Verification items for the finished model (mm, model axes). Give positions to 0.01 mm unless a question says otherwise; leave off trailing zeros. Write each loop counter-clockwise with the first axis right and the second up, starting at its lowest first coordinate (ties: lowest second). Pieces come first, ordered by that corner, then holes.
from build123d import *

# Parameters (mm, degrees)
EXTRUDE002_DEPTH = 3


with BuildPart() as axle_hex_extrude:
    # Sketch009 → Extrude002 (new body)
    with BuildSketch(Plane.YZ.offset(31)):
        Polygon((-48.5, -42.556624), (-51, -41.113249), (-53.5, -42.556624), (-53.5, -45.443376), (-51, -46.886751), (-48.5, -45.443376), align=None)
    extrude(amount=-EXTRUDE002_DEPTH)


with BuildPart() as axle_front:
    # Sketch008 → Revolve001 (revolve)
    with BuildSketch(Plane.XZ.offset(51)):
        with BuildLine():
            Line((27.5, -42.5), (-27.5, -42.5))
            Line((-27.5, -42.5), (-27.5, -37))
            Line((-27.5, -37), (-28, -37))
            ThreePointArc((-28, -37), (-29.86452, -40.281569), (-30.511358, -44))
            Line((-30.511358, -44), (30.511358, -44))
            ThreePointArc((30.511358, -44), (30.236308, -40.148184), (28, -37))
            Line((27.5, -37), (28, -37))
            Line((27.5, -42.5), (27.5, -37))
        make_face()
    revolve(axis=Axis((2, -51, -44), (1, 0, 0)))

    # Cut: cut axle-hex-extrude
    add(axle_hex_extrude.part, mode=Mode.SUBTRACT)


with BuildPart() as axle_back:
    # Part__Mirroring001: instance of axle-front
    add(axle_front.part.mirror(Plane(origin=(0, 0, 0), x_dir=(1, 0, 0), z_dir=(0, 1, 0))))


solid = axle_back.part
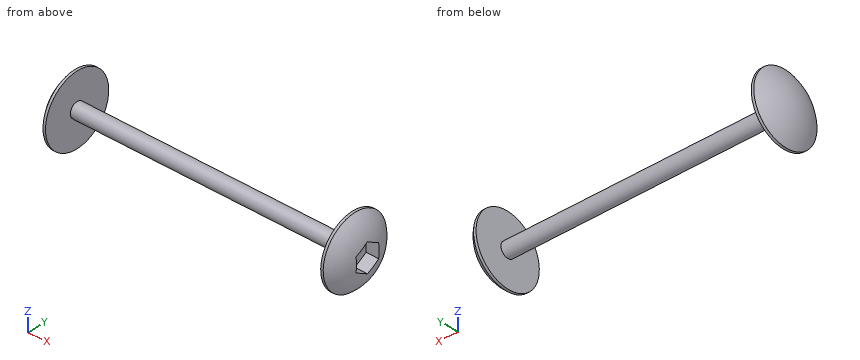
Item 1: Depth check by flat-ended pin: pin 1 (5 mm diameter, centred on x = 21, y = 53.5, fed in from +Z); pin 2 (5 mm diameter, centred on x = 21, z = -41.5, fed in from -Y); pin 3 (2 mm diameter, centred on y = 54.5, z = -48.5, fed in from -X). Enter the tip coordinate at first touch or a pass-through.
Answer key:
pin 1: stops at z = -42.5
pin 2: stops at y = 49.5
pin 3: stops at x = -29.46
Item 2: Sectioned sample at A-A on x = -20.5. Record the cut outline in (y, z).
Answer key:
outline: circle Ø3 at (51, -44)
Item 3: Scan lines: line 1 along X through (y, z) = (46.75, -39); line 2 along X through (y, z) = (50.25, -41); line 3 along Z through (x, y) = (-3.5, 51.75). Record each from-to range of solid material in increasing order.
Answer key:
line 1: x = -28.34 to -27.5, 27.5 to 28.49
line 2: x = -30.07 to -27.5, 27.5 to 30.46
line 3: z = -45.3 to -42.7
